```python
from build123d import *

# Parameters (mm, degrees)
ESBO_O1_W                = 3.8
ESBO_O1_H                = 45
RESSALTO_EXTRUS_O1_DEPTH = 3.8
ESBO_O2_R                = 1.5
RESSALTO_EXTRUS_O2_DEPTH = 10
ESBO_O3_W                = 2
ESBO_O3_H                = 3.8
RESSALTO_EXTRUS_O3_DEPTH = 1
ESBO_O5_R                = 1
CORTE_EXTRUS_O1_DEPTH    = 4
RESSALTO_EXTRUS_O7_DEPTH = 3.8
ESBO_O10_W               = 2
ESBO_O10_H               = 3.8
RESSALTO_EXTRUS_O8_DEPTH = 19


with BuildPart() as part:
    # Esboço1 → Ressalto-extrusão1 (new body)
    with BuildSketch(Plane.XY):
        with Locations((-14.624350205, 5.125)):
            Rectangle(ESBO_O1_W, ESBO_O1_H)
    extrude(amount=RESSALTO_EXTRUS_O1_DEPTH)

    # Esboço2 → Ressalto-extrusão2 (add)
    with BuildSketch(Plane.XY.offset(3.8)):
        with Locations((-14.624350205, -2.375)):
            Circle(ESBO_O2_R)
    extrude(amount=RESSALTO_EXTRUS_O2_DEPTH)

    # Esboço3 → Ressalto-extrusão3 (add)
    with BuildSketch(Plane(origin=(0, -17.375, 0), x_dir=(-1, 0, 0), z_dir=(0, -1, 0))):
        with Locations((13.724350205, -1.9)):
            Rectangle(ESBO_O3_W, ESBO_O3_H)
    extrude(amount=RESSALTO_EXTRUS_O3_DEPTH)

    # Esboço5 → Corte-extrusão1 (cut)
    with BuildSketch(Plane.XY.offset(3.8)):
        with Locations((-14.624350205, 12.625)):
            Circle(ESBO_O5_R)
    extrude(amount=-CORTE_EXTRUS_O1_DEPTH, mode=Mode.SUBTRACT)

    # Esboço9 → Ressalto-extrusão7 (add)
    with BuildSketch(Plane.XY.offset(3.8)):
        Polygon((-12.724350205, -18.375), (-12.724350205, -33.375), (-14.724350205, -33.375), (-16.524350205, -18.375), align=None)
    extrude(amount=-RESSALTO_EXTRUS_O7_DEPTH)

    # Esboço10 → Ressalto-extrusão8 (add)
    with BuildSketch(Plane(origin=(0, -33.375, 0), x_dir=(-1, 0, 0), z_dir=(0, -1, 0))):
        with Locations((13.724350205, -1.9)):
            Rectangle(ESBO_O10_W, ESBO_O10_H)
    extrude(amount=RESSALTO_EXTRUS_O8_DEPTH)


solid = part.part
```
Read the model definition and answer for the solid it produces. Units are mm, in the model's axes. A direction names the side the tool comes from. Coordinates: 2 decimals unless noted, no trailing zeros. Write each loop counter-clockwise with the first axis right and the second up, starting at its lowest first coordinate (ties: lowest second). Pieces come first, ordered by that corner, then holes. Notation, with made-up numbers: (28.5, -16) -> (62.5, -16) arc R32 cw to (62.5, 21) -> close; hole circle Ø3 at (2, 61.5). An arc over 180 degrees is marked (long way). Return JSON: item names as keys, results as strings.
1. Each of these flat-tipped pins is pushed along its axis until it touches: P1, Ø1.9, axis at x = -14.5, y = -29, coming from the +Z side; P2, Ø2, axis at x = -14.5, z = 7, coming from the -Y side (3 decimals); P3, Ø1.5, axis at y = -2.5, z = 11.5, coming from the -X side. Where does it stop, or does it pass through?
Found:
{"P1": "z = 3.8", "P2": "y = -3.875", "P3": "x = -16.12"}
2. Determine the mould class of faces 1 (the face through (-15.42, 12.02, 1.93)), 2 (the face through (-15, -3, 0)), 3 (the face through (-15.61, -25.98, 1.93)) for opening direction Y: pulls with the +Y half, pulls with the -Y half, needs draft (parallel to the pull), parting line crosses it, or undercut.
Found:
{"face 1": "undercut", "face 2": "needs draft", "face 3": "pulls with the -Y half"}
3. A cutting plane is placed at C-C (z = 11). Determine the outline of the cut face in (x, y) (3 decimals), and give its area (3 significant figures).
Found:
{"outline": "circle Ø3 at (-14.624, -2.375)", "area": "7.07 mm2"}
4. A cutting plane is placed at B-B (y = -7.5). Determine the outline of the cut face in (x, z), and give its area (3 significant figures).
Found:
{"outline": "(-16.52, 0) -> (-12.72, 0) -> (-12.72, 3.8) -> (-16.52, 3.8) -> close", "area": "14.4 mm2"}
5. A tool of negligible diameter and unlimited length cuts with its end or side. For faces 4 (the face through (-13.2, -1.9, 8.7)), 5 (the face through (-14.724, -43, 2)), 6 (the face through (-16, -18.375, 2)), 7 (the face through (-15, -2, 13.8)), from which of +Z, -Z, +X, -X, +Y, -Y can it reach the whole face along a straight path? Write none if from no direction.
Found:
{"face 4": "+Z", "face 5": "+Z, -Z, -X, -Y", "face 6": "+Z, -Z, -X", "face 7": "+Z, +X, -X, +Y, -Y"}
6. Find the intervals of material crossed by line 1 along Z through (x, y) = (-13.5, 22.5); line 2 along Y through (x, z) = (-13.8, 1.5) (3 decimals); line 3 along Y through (x, z) = (-15.1, 5), in increasing order. Write a range as from..to.
Found:
{"line 1": "0..3.8", "line 2": "-52.375..12.059, 13.191..27.625", "line 3": "-3.8..-0.95"}
7. A cutting plane is placed at D-D (y = -38). Determine the outline of the cut face in (x, z).
Found:
{"outline": "(-14.72, 0) -> (-12.72, 0) -> (-12.72, 3.8) -> (-14.72, 3.8) -> close"}
8. A cutting plane is placed at A-A (z = 3). Determine the outline of the cut face in (x, y) (3 decimals), and give its area (3 significant figures).
Found:
{"outline": "(-16.524, -18.375) -> (-14.724, -33.375) -> (-14.724, -52.375) -> (-12.724, -52.375) -> (-12.724, 27.625) -> (-16.524, 27.625) -> (-16.524, -17.375) -> (-14.724, -17.375) -> (-14.724, -18.375) -> close; hole circle Ø2 at (-14.624, 12.625)", "area": "251 mm2"}
